from build123d import *

# Parameters (mm, degrees)
SKETCH_1_W          = 105
SKETCH_1_H          = 180
EXTRUDE_1_DEPTH     = 3
CUT_EXTRUDE_1_DEPTH = 10
SKETCH_3_R          = 3
CUT_EXTRUDE_2_DEPTH = 2
SKETCH_4_R          = 1.425
CUT_EXTRUDE_3_DEPTH = 2


with BuildPart() as part:
    # Эскиз1 → Бобышка-Вытянуть1 (new body)
    with BuildSketch(Plane.XY):
        Rectangle(SKETCH_1_W, SKETCH_1_H)
    extrude(amount=EXTRUDE_1_DEPTH)

    # Эскиз2 → Вырез-Вытянуть1 (cut)
    with BuildSketch(Plane(origin=(0, 0, 0), x_dir=(-1, 0, 0), z_dir=(0, 0, -1))):
        with BuildLine():
            Line((-26.25, -44), (-26.25, -46))
            ThreePointArc((-26.25, -46), (-25.298097039, -48.298097039), (-23, -49.25))
            Line((-23, -49.25), (-22.75, -49.25))
            ThreePointArc((-22.75, -49.25), (-15.678932188, -52.178932188), (-12.75, -59.25))
            Line((-12.75, -59.25), (-12.75, -79.25))
            ThreePointArc((-12.75, -79.25), (-12.164213562, -80.664213562), (-10.75, -81.25))
            Line((-10.75, -81.25), (10.75, -81.25))
            ThreePointArc((10.75, -81.25), (12.164213562, -80.664213562), (12.75, -79.25))
            Line((12.75, -79.25), (12.75, -59.25))
            ThreePointArc((12.75, -59.25), (15.678932188, -52.178932188), (22.75, -49.25))
            Line((22.75, -49.25), (23, -49.25))
            ThreePointArc((23, -49.25), (25.298097039, -48.298097039), (26.25, -46))
            Line((26.25, -46), (26.25, -44))
            ThreePointArc((26.25, -44), (25.298097039, -41.701902961), (23, -40.75))
            Line((23, -40.75), (-23, -40.75))
            ThreePointArc((-23, -40.75), (-25.298097039, -41.701902961), (-26.25, -44))
        make_face()
    extrude(amount=-CUT_EXTRUDE_1_DEPTH, mode=Mode.SUBTRACT)

    # Эскиз3 → Вырез-Вытянуть2 (cut)
    with BuildSketch(Plane.XY.offset(3)):
        with Locations((-50.5, 88)):
            Circle(SKETCH_3_R)
        with Locations((0, 88)):
            Circle(SKETCH_3_R)
        with Locations((50.5, 88)):
            Circle(SKETCH_3_R)
        with Locations((50.5, 0)):
            Circle(SKETCH_3_R)
        with Locations((50.5, -88)):
            Circle(SKETCH_3_R)
        with Locations((0, -88)):
            Circle(SKETCH_3_R)
        with Locations((-50.5, -88)):
            Circle(SKETCH_3_R)
        with Locations((-50.5, 0)):
            Circle(SKETCH_3_R)
    extrude(amount=-CUT_EXTRUDE_2_DEPTH, mode=Mode.SUBTRACT)

    # Эскиз4 → Вырез-Вытянуть3 (cut)
    with BuildSketch(Plane.XY.offset(1)):
        with Locations((-50.5, 88)):
            Circle(SKETCH_4_R)
        with Locations((0, 88)):
            Circle(SKETCH_4_R)
        with Locations((50.5, 88)):
            Circle(SKETCH_4_R)
        with Locations((50.5, 0)):
            Circle(SKETCH_4_R)
        with Locations((50.5, -88)):
            Circle(SKETCH_4_R)
        with Locations((0, -88)):
            Circle(SKETCH_4_R)
        with Locations((-50.5, -88)):
            Circle(SKETCH_4_R)
        with Locations((-50.5, 0)):
            Circle(SKETCH_4_R)
    extrude(amount=-CUT_EXTRUDE_3_DEPTH, mode=Mode.SUBTRACT)


solid = part.part
Verification items for the finished model (mm, model axes). A direction names the side the tool comes from. Coordinates: 2 decimals unless noted, no trailing zeros. Order: outer loops, then holes, each group sorted by start corner. A loop starts at its lowest first (then second) coordinate and runs counter-clockwise, first axis right, second up.
1. Release check for a two-part mould opening along Y. For faces 1 (the face through (0, -86, 1)), 2 (the face through (-1, 1, 0)), 3 (the face through (-47.5, -0.1, 2)) record: +Y half, -Y half, draft (parallel to the pull), parting line (faces both ways), or undercut.
Results found:
face 1: undercut
face 2: draft
face 3: undercut
2. Set-up check for faces 4 (the face through (-48.9, 0, 1)), 5 (the face through (15.76, -52.1, 1.48)): record each of +Z, -Z, +X, -X, +Y, -Y from which the full face is reachable in a straight line by a thin tool's end or side.
Results found:
face 4: +Z
face 5: +Z, -Z
3. Scan lines: line 1 (Y direction, x = 0, z = 0.7) (3 decimals); line 2 (Y direction, x = 11, z = 1.5); line 3 (X direction, y = 88, z = 0.6) (3 decimals). Record each from-to range of solid material in increasing order.
Results found:
line 1: y = -90 to -89.425, -86.575 to -81.25, -40.75 to 86.575, 89.425 to 90
line 2: y = -90 to -81.23, -40.75 to 90
line 3: x = -52.5 to -51.925, -49.075 to -1.425, 1.425 to 49.075, 51.925 to 52.5
4. Sectioned sample at B-B, the plane y = -77. Record the cut outline in (x, z).
Results found:
outline: (-52.5, 0) - (-12.75, 0) - (-12.75, 3) - (-52.5, 3) - close; (12.75, 0) - (52.5, 0) - (52.5, 3) - (12.75, 3) - close
5. Sectioned sample at A-A, the plane x = 5.5. Record the cut outline in (y, z).
Results found:
outline: (-90, 0) - (-81.25, 0) - (-81.25, 3) - (-90, 3) - close; (-40.75, 0) - (90, 0) - (90, 3) - (-40.75, 3) - close
6. Go/stop test with a flat-tipped pin: pin 1 Ø3.5 at (x, y) = (50.5, -88) entering from +Z. Record where the tip stops, or that it passes through.
Results found:
pin 1: stops at z = 1
